Read the model definition and answer for the solid it produces. Units are mm, in the model's axes. Face numbers are marked on the shaded views. A direction names the side the tool comes from. Give positions to 0.01 mm unless a question says otherwise; leave off trailing zeros. Loops run counter-clockwise (first coordinate to the right, second up) from the corner with the lowest first, then second, coordinate; pieces in that order, holes last. Notation, with made-up numbers: (30, -0.5) - (72, -0.5) arc R27 cw to (72, 23.5) - close; hole circle Ø8 at (7, 5). An arc over 180 degrees is marked (long way). Put each result on its own line as item: value. Start each with the question number.
1. For a pull along Y with two mould halves and no side action, classify the marked faces 3, 4, 5 and 6 as released by +Y, released by -Y, zero draft, split by the parting line, or undercut.
2. A cutting plane is placed at D-D, the plane z = 5.5. Determine the outline of the cut face in (x, y), plus the area to 3 significant figures.
3. A cutting plane is placed at B-B, the plane x = 1.6. Determine the outline of the cut face in (y, z), plus the area to 3 significant figures.
4. Consider L1, parallel to Z at x = -1.6, y = 16; L2, parallel to X at y = 5.5, z = 4; L3, parallel to Y at x = 0.3, z = 3.75. Determine where each line is inside the solid, lowest interval first. Write a range as from..to.
5. A cutting plane is placed at A-A, the plane z = 0.5. Determine the outline of the cut face in (x, y), plus the area to 3 significant figures.
6. For the marked faces 1 and 2, determine the directions among +Z, -Z, +X, -X, +Y, -Y from which every point of the face is accessible in a straight line to the end or side of a thin tool.
7. Given pin 1 Ø1 at (x, z) = (1.5, 5.5) entering from -Y; pin 2 Ø3 at (y, z) = (4, 4.5) entering from -X; pin 3 Ø1.5 at (x, y) = (-1.5, 17) entering from -Z; pin 4 Ø2.5 at (x, y) = (-1.5, 18.5) entering from +Z, each flat-ended and moving along its own axis, determine where each tip first touches the part or whether it passes through.
8. A cutting plane is placed at C-C, the plane y = 6.25. Determine the outline of the cut face in (x, z).
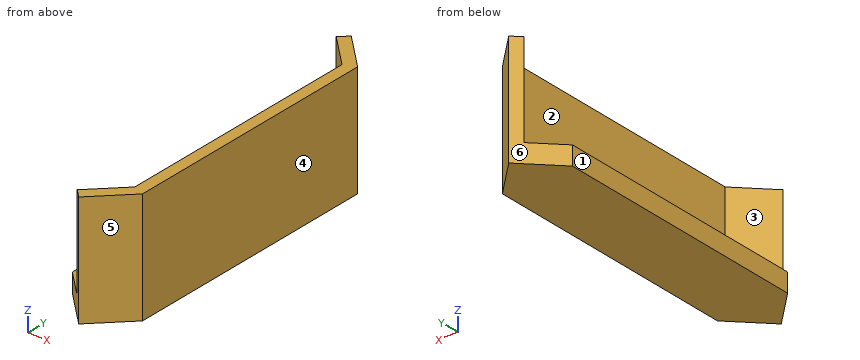
```python
from build123d import *

# Parameters (mm, degrees)
EXTRUDE_1_DEPTH     = 1.6
EXTRUDE_2_DEPTH     = 8
CUT_EXTRUDE_1_DEPTH = 8


with BuildPart() as part:
    # 草图1 → 凸台-拉伸1 (new body)
    with BuildSketch(Plane.XY):
        Polygon((0, 0), (-3, 3), (-3, 25.5), (0, 28.5), (3, 25.5), (3, 3), align=None)
    extrude(amount=EXTRUDE_1_DEPTH)

    # 草图2 → 凸台-拉伸2 (add)
    with BuildSketch(Plane.XY.offset(1.6)):
        Polygon((0, 0), (3, 3), (3, 25.5), (0, 28.5), (-3, 25.5), (-3, 3), align=None)
        Polygon((0, 1.414213562), (2, 3.414213562), (2, 25.085786438), (0, 27.085786438), (-2, 25.085786438), (-2, 3.414213562), align=None, mode=Mode.SUBTRACT)
    extrude(amount=EXTRUDE_2_DEPTH)

    # 草图3 → 切除-拉伸1 (cut)
    with BuildSketch(Plane.XY.offset(9.6)):
        Polygon((0, 27.085786438), (-0.707106781, 27.792893219), (-3, 25.5), (-3, 3), (-0.707106781, 0.707106781), (0, 1.414213562), (-2, 3.414213562), (-2, 25.085786438), align=None)
    extrude(amount=-CUT_EXTRUDE_1_DEPTH, mode=Mode.SUBTRACT)


solid = part.part
```
Return value:
1. face 3: undercut
1. face 4: zero draft
1. face 5: released by -Y
1. face 6: released by +Y
2. outline: (-0.71, 0.71) - (0, 0) - (3, 3) - (3, 25.5) - (0, 28.5) - (-0.71, 27.79) - (2, 25.09) - (2, 3.41) - close
2. area: 30.2 mm2
3. outline: (1.6, 0) - (26.9, 0) - (26.9, 9.6) - (25.49, 9.6) - (25.49, 1.6) - (3.01, 1.6) - (3.01, 9.6) - (1.6, 9.6) - close
3. area: 63.1 mm2
4. L1: z = 0..1.6
4. L2: x = 2..3
4. L3: y = 0.3..1.71, 26.79..28.2
5. outline: (-3, 3) - (0, 0) - (3, 3) - (3, 25.5) - (0, 28.5) - (-3, 25.5) - close
5. area: 153 mm2
6. face 1: +Z, -Z, -X, +Y, -Y
6. face 2: +Z, -X
7. pin 1: stops at y = 1
7. pin 2: stops at x = 1.09
7. pin 3: stops at z = 0
7. pin 4: stops at z = 1.6
8. outline: (-3, 0) - (3, 0) - (3, 9.6) - (2, 9.6) - (2, 1.6) - (-3, 1.6) - close
